Verification items for the finished model (mm, model axes). A direction names the side the tool comes from. Coordinates: 2 decimals unless noted, no trailing zeros. Order: outer loops, then holes, each group sorted by start corner. A loop starts at its lowest first (then second) coordinate and runs counter-clockwise, first axis right, second up.
Q1. Depth check by flat-ended pin: P1, Ø2, axis at x = 1, z = 4, coming from the -Y side; P2, Ø4, axis at y = -7, z = 2, coming from the -X side; P3, Ø4, axis at x = 10.5, z = 1.5, coming from the -Y side. Enter the tip coordinate at first touch or a pass-through.
Q2. Cross-section at C-C, the plane x = 11. Count the separate pieces of the cut face and the enclosed holes in it, and give its area (3 significant figures).
Q3. Draft check along Y on faces 1 (the cylindrical face through (-0.806, 6.914, 5.265)), 2 (the cylindrical face through (17.565, 1.254, -0.479)). Enter one of: pulls with the +Y half, pulls with the -Y half, needs draft (parallel to the pull), parting line crosses it, or undercut.
Q4. Cross-section at A-A, the plane y = 0. Record the boundary of the cut face in (x, z), and give its area (3 significant figures).
Q5. Set-up check for faces 3 (the flat face through (1.3, 7.9, 2.6)), 4 (the cylindrical face through (-0.544, 17.722, -0.479)), 5 (the cylindrical face through (-1.43, 3.04, 4.45)): record each of +Z, -Z, +X, -X, +Y, -Y from which the full face is reachable in a straight line by a thin tool's end or side.
Q6. Cross-section at B-B, the plane z = 4. Record the boundary of the cut face in (x, y) (3 decimals).
Q7. Thickness scan on line 1 (X direction, y = 0, z = 4.5); line 2 (Y direction, x = -8.5, z = 0); line 3 (Z direction, x = 0, y = 7). Record the ranges inside material, lowest first.
from build123d import *

# Parameters (mm, degrees)
F0_R     = 2.75
F0_W     = 5.75
F0_H     = 2.4
F1_DEPTH = 7
F4_R     = 4.1752398448
F5_DEPTH = 3.001
F6_R     = 1.5
F7_DEPTH = 6.595113986


with BuildPart() as f1:
    # F0 (on Top) → F1 (new body)
    with BuildSketch(Plane.XY):
        with BuildLine():
            Line((2.875, 7.9), (-2.875, 7.9))
            ThreePointArc((-2.875, 7.9), (0, -8.4068796233), (2.875, 7.9))
        make_face()
        Circle(F0_R, mode=Mode.SUBTRACT)
        with Locations((0, 4.7)):
            Rectangle(F0_W, F0_H, mode=Mode.SUBTRACT)
    extrude(amount=F1_DEPTH)

    # F2 (on Front) → F3 (revolve)
    with BuildSketch(Plane.XZ):
        Polygon((0, 1), (0, 0), (0, -2), (25, -2), (22.8786796564, 0.1213203436), (25, 2.2426406871), (20, 2.2426406871), (18.7573593129, 1), align=None)
    revolve(axis=Axis((0, 0, -1), (0, 0, 1)))

    # F4 (on face) → F5 (cut, through all)
    with BuildSketch(Plane.XY.offset(1)):
        with Locations((13.5821194681, 0)):
            Circle(F4_R)
        with Locations((9.6040087788, -9.6040087788)):
            Circle(F4_R)
        with Locations((0, -13.5821194681)):
            Circle(F4_R)
        with Locations((-9.6040087788, -9.6040087788)):
            Circle(F4_R)
        with Locations((-13.5821194681, 0)):
            Circle(F4_R)
        with Locations((-9.6040087788, 9.6040087788)):
            Circle(F4_R)
        with Locations((0, 13.5821194681)):
            Circle(F4_R)
        with Locations((9.6040087788, 9.6040087788)):
            Circle(F4_R)
    extrude(amount=-F5_DEPTH, mode=Mode.SUBTRACT)

    # F6 (on face) → F7 (cut, up to face)
    with BuildSketch(Plane(origin=(0, 7.9, 0), x_dir=(-1, 0, 0), z_dir=(0, 1, 0))):
        with Locations((0, 4)):
            Circle(F6_R)
    extrude(amount=-F7_DEPTH, mode=Mode.SUBTRACT)


solid = f1.part
Check values:
1. P1: stops at y = -8.41
1. P2: stops at x = -24.49
1. P3: stops at y = -23.46
2. separate pieces: 4
2. enclosed holes: 0
2. area: 73.8 mm2
3. face 1: needs draft
3. face 2: undercut
4. outline: (-25, -2) - (-17.76, -2) - (-17.76, 1) - (-18.76, 1) - (-20, 2.24) - (-25, 2.24) - (-22.88, 0.12) - close; (-9.41, -2) - (9.41, -2) - (9.41, 1) - (8.41, 1) - (8.41, 7) - (2.75, 7) - (2.75, 1) - (-2.75, 1) - (-2.75, 7) - (-8.41, 7) - (-8.41, 1) - (-9.41, 1) - close; (17.76, -2) - (25, -2) - (22.88, 0.12) - (25, 2.24) - (20, 2.24) - (18.76, 1) - (17.76, 1) - close
4. area: 173 mm2
5. face 3: +Z
5. face 4: +Z, -Z
5. face 5: +Y
6. outline: (-2.875, 3.5) - (-2.875, 5.9) - (-1.5, 5.9) - (-1.5, 7.9) - (-2.875, 7.9) arc R8.407 ccw (long way) to (2.875, 7.9) - (1.5, 7.9) - (1.5, 5.9) - (2.875, 5.9) - (2.875, 3.5) - (1.5, 3.5) - (1.5, 2.305) arc R2.75 cw (long way) to (-1.5, 2.305) - (-1.5, 3.5) - close
7. line 1: x = -8.41 to -2.75, 2.75 to 8.41
7. line 2: y = -21.37 to -13.63, -5.58 to 5.58, 13.63 to 21.37
7. line 3: z = -2 to 2.5, 5.5 to 7
